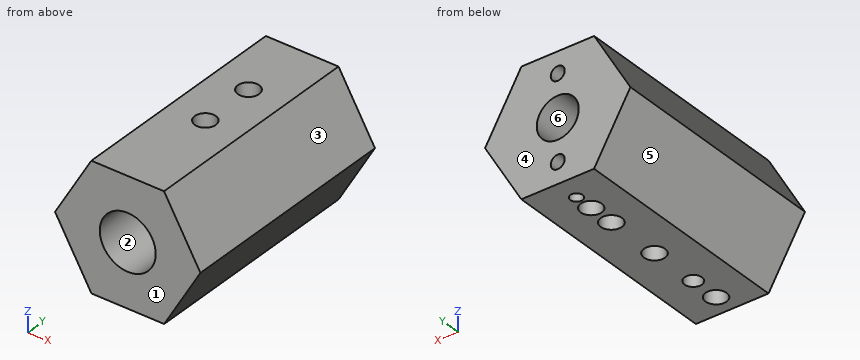
from build123d import *

# Parameters (mm, degrees)
F1_DEPTH  = 65
F2_R      = 6
F3_DEPTH  = 65
F4_R      = 3.0447564862
F5_DEPTH  = 36
F6_R      = 3.0186568284
F7_DEPTH  = 36
F8_R      = 1.75
F9_DEPTH  = 14
F10_R     = 2.5
F11_DEPTH = 14
F12_R     = 8
F12_R_2   = 6
F13_DEPTH = 19
F16_D     = 4
F16_DEPTH = 12
F16_TIP   = 1.2017212381
F18_D     = 4
F18_DEPTH = 12
F18_TIP   = 1.2017212381
F20_D     = 6
F20_DEPTH = 8
F20_TIP   = 1.8025818571
F22_D     = 6
F22_DEPTH = 10
F22_TIP   = 1.8025818571


with BuildPart() as f1:
    # F0 (on Front) → F1 (new body)
    with BuildSketch(Plane.XZ):
        Polygon((10.4105382668, -17.9894606088), (20.784599021, 0.0210603017), (10.3740607542, 18.0105209105), (-10.4105382668, 17.9894606088), (-20.784599021, -0.0210603017), (-10.3740607542, -18.0105209105), align=None)
    extrude(amount=F1_DEPTH)

    # F2 (on face) → F3 (cut)
    with BuildSketch(Plane.XZ.offset(65)):
        Circle(F2_R)
    extrude(amount=-F3_DEPTH, mode=Mode.SUBTRACT)

    # F4 (on face) → F5 (cut)
    with BuildSketch(Plane(origin=(-0.0182387563, 0, 17.9999907597), x_dir=(0.9999994866, 0, 0.0010132642), z_dir=(-0.0010132642, 0, 0.9999994866))):
        with Locations((0, -20.0090762228)):
            Circle(F4_R)
    extrude(amount=-F5_DEPTH, mode=Mode.SUBTRACT)

    # F6 (on face) → F7 (cut)
    with BuildSketch(Plane(origin=(-0.0182387563, 0, 17.9999907597), x_dir=(0.9999994866, 0, 0.0010132642), z_dir=(-0.0010132642, 0, 0.9999994866))):
        with Locations((0, -36.0637567937)):
            Circle(F6_R)
    extrude(amount=-F7_DEPTH, mode=Mode.SUBTRACT)

    # F8 (on face) → F9 (cut)
    with BuildSketch(Plane(origin=(0.0182387563, 0, -17.9999907597), x_dir=(0.9999994866, 0, 0.0010132642), z_dir=(0.0010132642, 0, -0.9999994866))):
        with Locations((0, 7)):
            Circle(F8_R)
    extrude(amount=-F9_DEPTH, mode=Mode.SUBTRACT)

    # F10 (on face) → F11 (cut)
    with BuildSketch(Plane(origin=(0.0182387563, 0, -17.9999907597), x_dir=(0.9999994866, 0, 0.0010132642), z_dir=(0.0010132642, 0, -0.9999994866))):
        with Locations((0, 50.5)):
            Circle(F10_R)
    extrude(amount=-F11_DEPTH, mode=Mode.SUBTRACT)

    # F12 (on face) → F13 (cut)
    with BuildSketch(Plane.XZ.offset(65)):
        Circle(F12_R)
        Circle(F12_R_2, mode=Mode.SUBTRACT)
    extrude(amount=-F13_DEPTH, mode=Mode.SUBTRACT)

    # F16
    with Locations(Plane(origin=(0, 0, 0), x_dir=(-1, 0, 0), z_dir=(0, 1, 0))):
        with Locations((0, 12)):
            Hole(F16_D / 2, depth=F16_DEPTH)
            with Locations((0, 0, -(F16_DEPTH + F16_TIP / 2))):  # 118° drill point
                Cone(0, F16_D / 2, F16_TIP, mode=Mode.SUBTRACT)

    # F18
    with Locations(Plane(origin=(0, 0, 0), x_dir=(-1, 0, 0), z_dir=(0, 1, 0))):
        with Locations((0, -12)):
            Hole(F18_D / 2, depth=F18_DEPTH)
            with Locations((0, 0, -(F18_DEPTH + F18_TIP / 2))):  # 118° drill point
                Cone(0, F18_D / 2, F18_TIP, mode=Mode.SUBTRACT)

    # F20
    with Locations(Plane(origin=(0.0182387563, 0, -17.9999907597), x_dir=(0.9999994866, 0, 0.0010132642), z_dir=(0.0010132642, 0, -0.9999994866))):
        with Locations((0, 59)):
            Hole(F20_D / 2, depth=F20_DEPTH)
            with Locations((0, 0, -(F20_DEPTH + F20_TIP / 2))):  # 118° drill point
                Cone(0, F20_D / 2, F20_TIP, mode=Mode.SUBTRACT)

    # F22
    with Locations(Plane(origin=(0.0182387563, 0, -17.9999907597), x_dir=(0.9999994866, 0, 0.0010132642), z_dir=(0.0010132642, 0, -0.9999994866))):
        with Locations((0, 12.5)):
            Hole(F22_D / 2, depth=F22_DEPTH)
            with Locations((0, 0, -(F22_DEPTH + F22_TIP / 2))):  # 118° drill point
                Cone(0, F22_D / 2, F22_TIP, mode=Mode.SUBTRACT)


solid = f1.part
Source: CAD feature listing. Evaluate the final solid. Frame: model axes, mm. Face numbers are marked on the shaded views. A direction names the side the tool comes from. Round coordinates to 2 decimals unless told otherwise and drop trailing zeros. Loops run counter-clockwise (first coordinate to the right, second up) from the corner with the lowest first, then second, coordinate; pieces in that order, holes last. Notation, with made-up numbers: M 66,50.5 L 73,50.5 A26 ccw 73,75.5 Z; hole C -7,69 d1. An arc over 180 degrees is marked long. Return JSON: item names as keys, results as strings. Group by question number.
1. Section query C-C on x = -4.5. Output: boundary loops of the cut face in (y, z), and give its area (3 significant figures).
2. Section query B-B on z = -1.5. Output: boundary loops of the cut face in (x, y).
3. Pin query (flat end, axial travel): pin 1 (5 mm diameter, centred on x = 5, y = -23.5, fed in from -Z); pin 2 (6 mm diameter, centred on x = 15, y = -36.5, fed in from +Z); pin 3 (14 mm diameter, centred on x = 0, z = 0, fed in from -Y). Return the tip coordinate at first contact, or that it passes through.
4. Material intervals for line 1 along Z through (x, y) = (0, -28.5); line 2 along X through (y, z) = (-19, 5); line 3 along X through (y, z) = (-14, 2), sorted ascending. Write a range as from..to.
5. Reachability of the marked faces 1 and 2 from +Z, -Z, +X, -X, +Y, -Y: full face, straight path, thin tool, end or side. Return the list, or none.
6. Section query A-A on y = -41.5. Output: boundary loops of the cut face in (x, z).
7. Mould query, pull axis Z, two halves, no side actions, for the marked faces 3, 4, 5 and 6. Classes: released by +Z, released by -Z, zero draft, split by the parting line, or undercut.
8. Section query D-D on z = -12. State how many separate pieces and enclosed holes the cut face has, and give its area (3 significant figures).
Checks:
{
 "1": {"outline": "M -65,-18 L 0,-18 L 0,-3.97 L -46,-3.97 L -46,-6.61 L -65,-6.61 Z; M -65,6.61 L -46,6.61 L -46,3.97 L 0,3.97 L 0,18 L -65,18 Z", "area": "1,720 mm²"},
 "2": {"outline": "M -19.93,-65 L -7.86,-65 L -7.86,-46 L -5.81,-46 L -5.81,0 L -19.93,0 Z; M 5.81,-46 L 7.86,-46 L 7.86,-65 L 19.91,-65 L 19.91,0 L 5.81,0 Z"},
 "3": {"pin 1": "stops at z = -18", "pin 2": "stops at z = 15.2", "pin 3": "stops at y = -46"},
 "4": {"line 1": "z = -18..-6, 6..18", "line 2": "x = -17.89..-3.32, 3.32..17.9", "line 3": "x = -19.62..-5.66, 5.66..19.64"},
 "5": {"face 1": "+Z, -Z, +X, -X, -Y", "face 2": "-Y"},
 "6": {"outline": "M -20.78,-0.02 L -10.37,-18.01 L 10.41,-17.99 L 20.78,0.02 L 10.37,18.01 L -10.41,17.99 Z; hole C 0,0 d12"},
 "7": {"face 3": "released by +Z", "face 4": "zero draft", "face 5": "released by -Z", "face 6": "undercut"},
 "8": {"separate pieces": "1", "enclosed holes": "4", "area": "1,630 mm²"}
}
